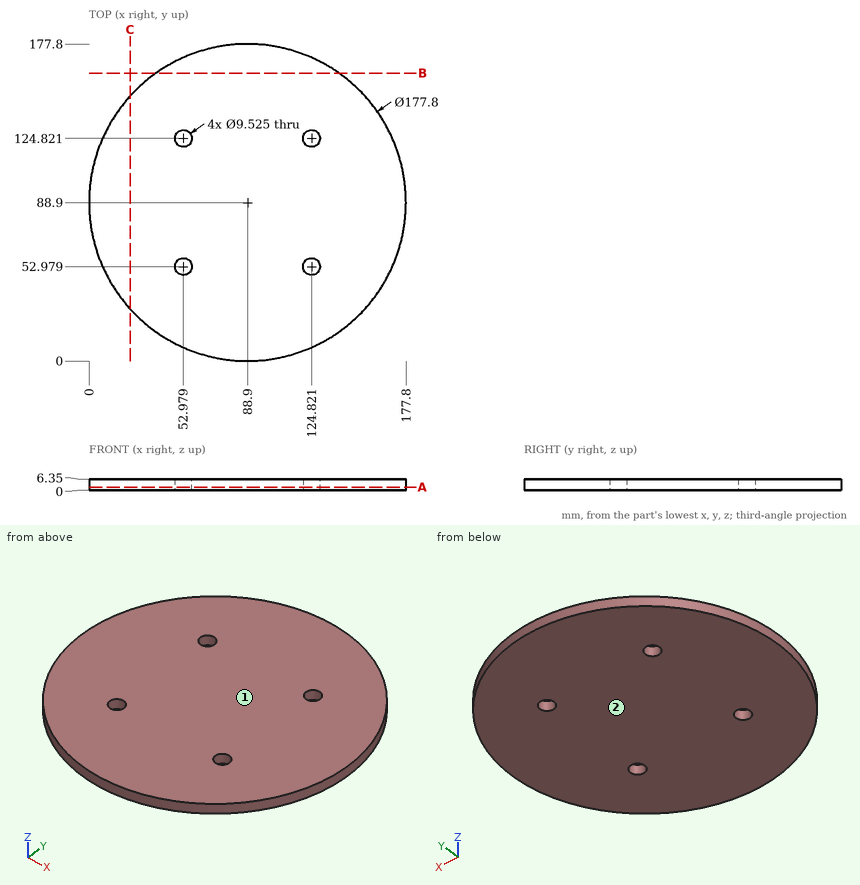
Source: three-view drawing plus pictorial views. Frame: mm from the lowest corner of the part. Round coordinates to 2 decimals unless told otherwise and drop trailing zeros. Write each loop counter-clockwise with the first axis right and the second up, starting at its lowest first coordinate (ties: lowest second). Pieces come first, ordered by that corner, then holes. Notation, with made-up numbers: M 64,30 L 73,30 A21 cw 73,36 Z; hole C 57.5,77.5 d4. An arc over 180 degrees is marked long. Write each question's results on one line, items separated by ' | '.
Q1. Pin query (flat end, axial travel): P1, Ø3, axis at y = 145, z = 3.5, coming from the -X side; P2, Ø1, axis at x = 136, z = 1, coming from the -Y side; P3, Ø1, axis at y = 115.5, z = 2, coming from the +X side. Return the tip coordinate at first contact, or that it passes through.
Results:
P1: stops at x = 18.74 | P2: stops at y = 13.19 | P3: stops at x = 173.88
Q2. Section query C-C (x = 23). Return loops of the section in (y, z).
Results:
outline: M 29.23,0 L 148.57,0 L 148.57,6.35 L 29.23,6.35 Z
Q3. Draft query along Z for the marked faces 1 and 2. Return one class per face: released by +Z, released by -Z, zero draft, split by the parting line, or undercut.
Results:
face 1: released by +Z | face 2: released by -Z
Q4. Section query B-B (y = 161.5). Return loops of the section in (x, z), and give its area (3 significant figures).
Results:
outline: M 37.59,0 L 140.21,0 L 140.21,6.35 L 37.59,6.35 Z | area: 652 mm^2
Q5. Line query: line 1 along Y through (x, z) = (128, 3.5); line 2 along Y through (x, z) = (126.5, 5); line 3 along X through (y, z) = (53, 3). Output: solid intervals per line, ascending.
Results:
line 1: y = 9.06 to 49.43, 56.53 to 121.27, 128.37 to 168.74 | line 2: y = 8.34 to 48.52, 57.44 to 120.36, 129.28 to 169.46 | line 3: x = 7.57 to 48.22, 57.74 to 120.06, 129.58 to 170.23
Q6. Section query A-A (z = 1.75). Return loops of the section in (x, y) (1 decimal), and give its area (3 significant figures).
Results:
outline: C 88.9,88.9 d177.8; hole C 53,53 d9.5; hole C 53,124.8 d9.5; hole C 124.8,53 d9.5; hole C 124.8,124.8 d9.5 | area: 24,500 mm^2
